Input: part model. Units: mm. Frame: model coordinates. A direction names the side the tool comes from. Coordinates: 2 decimals unless noted, no trailing zeros. Write each loop counter-clockwise with the first axis right and the second up, starting at its lowest first coordinate (ties: lowest second). Pieces come first, ordered by that corner, then holes. Notation, with made-up numbers: (89, 2) - (101, 2) arc R13 cw to (101, 17) - close; hole circle Ø6 at (-1, 23). An arc over 180 degrees is marked (long way). Put each result on its own line as item: value. Start each with the question number.
1. Cut plane C-C, the plane y = 0. Count the separate pieces of the cut face and the enclosed holes in it, and give its area (3 significant figures).
2. Access query for faces 1 (the cylindrical face through (23.82, -1.53, 8.77)), 2 (the flat face through (-16, 0, 17.78)), 3 (the cylindrical face through (12.114, 3.815, 28.4)), 4 (the flat face through (-43, 12.7, 13)). Directions: +Z, -Z, +X, -X, +Y, -Y. A direction counts if a zero-diameter tool reaches every point of the face in a straight line with its end or side. Return the directions, or none.
3. Pull-direction query (X, two-part tool) for faces 5 (the cylindrical face through (0.372, 25.397, 12.878)), 6 (the flat face through (-42, 10.16, 13)), 7 (the flat face through (0, 8.89, 11)); classes: released by +X, released by -X, zero draft, split by the parting line, or undercut.
4. Pin query (flat end, axial travel): pin 1 (10 mm diameter, centred on x = -37.5, y = 2.5, fed in from +Z); pin 2 (1.5 mm diameter, centred on x = 10.5, z = 9.5, fed in from -Y); pin 3 (2 mm diameter, centred on x = 42, y = -0.5, fed in from -Z); pin 4 (12 mm diameter, centred on y = 0.5, z = 7.5, fed in from +X). Return the tip coordinate at first contact, or that it passes through.
5. Cut plane D-D, the plane y = 7. Return loops of the section in (x, z).
6. Line query: line 1 (Y direction, x = 0, z = 19); line 2 (Y direction, x = -41, z = 9); line 3 (X direction, y = 0, z = 25). Output: solid intervals per line, ascending.
7. Cut plane B-B, the plane x = 0. Return loops of the section in (y, z), and give its area (3 significant figures).
8. Cut plane A-A, the plane z = 5. Return loops of the section in (x, y), and give its area (3 significant figures).
from build123d import *

# Parameters (mm, degrees)
F0_W      = 127
F0_H      = 25.4
F1_DEPTH  = 25.4
F2_T      = -2.54
F3_R      = 25.4
F4_DEPTH  = 25.4
F5_R      = 19.05
F6_DEPTH  = 12.7
F7_R      = 12.7
F8_DEPTH  = 25.4
F9_W      = 17.78
F9_H      = 17.78
F10_DEPTH = 150.622
F11_W     = 40.64
F11_H     = 10.16
F12_DEPTH = 12.7
F13_R     = 5.528236
F13_R_2   = 5.08
F14_DEPTH = 17.78


with BuildPart() as f1:
    # F0 (on Top) → F1 (new body)
    with BuildSketch(Plane.XY):
        Rectangle(F0_W, F0_H)
    extrude(amount=F1_DEPTH)

    # F2
    f2_openings = [f1.faces().sort_by_distance(p)[0] for p in [
        (63.5, 0, 12.7),
    ]]
    offset(amount=F2_T, openings=f2_openings)

    # F3 (on face) → F4 (join)
    with BuildSketch(Plane.XY.offset(25.4)):
        Circle(F3_R)
    extrude(amount=-F4_DEPTH)

    # F5 (on face) → F6 (join)
    with BuildSketch(Plane.XY.offset(25.4)):
        Circle(F5_R)
    extrude(amount=F6_DEPTH)

    # F7 (on face) → F8 (cut)
    with BuildSketch(Plane.XY.offset(38.1)):
        Circle(F7_R)
    extrude(amount=-F8_DEPTH, mode=Mode.SUBTRACT)

    # F9 (on face) → F10 (cut)
    with BuildSketch(Plane(origin=(-63.5, 0, 0), x_dir=(0, -1, 0), z_dir=(-1, 0, 0))):
        with Locations((0, 12.7)):
            Rectangle(F9_W, F9_H)
    extrude(amount=-F10_DEPTH, mode=Mode.SUBTRACT)

    # F11 (on face) → F12 (cut)
    with BuildSketch(Plane(origin=(0, 0, 0), x_dir=(1, 0, 0), z_dir=(0, 0, -1))):
        with Locations((-36.008236, 0)):
            Rectangle(F11_W, F11_H)
        with Locations((39.295297, 0)):
            Rectangle(F11_W, F11_H)
    extrude(amount=-F12_DEPTH, mode=Mode.SUBTRACT)

    # F13 (on face) → F14 (join)
    with BuildSketch(Plane(origin=(0, 0, 0), x_dir=(1, 0, 0), z_dir=(0, 0, -1))):
        with Locations((-15.688236, 0)):
            Circle(F13_R)
        with Locations((18.975297, 0)):
            Circle(F13_R_2)
    extrude(amount=-F14_DEPTH)


solid = f1.part
Report:
1. separate pieces: 5
1. enclosed holes: 0
1. area: 955 mm^2
2. face 1: none
2. face 2: +X, -X
2. face 3: +Z
2. face 4: +Z, -Z, -X, +Y
3. face 5: split by the parting line
3. face 6: undercut
3. face 7: zero draft
4. pin 1: stops at z = 25.4
4. pin 2: stops at y = -23.45
4. pin 3: stops at z = 22.86
4. pin 4: stops at x = 63.5
5. outline: (-63.5, 0) - (63.5, 0) - (63.5, 2.54) - (24.42, 2.54) - (24.42, 3.81) - (-24.42, 3.81) - (-24.42, 2.54) - (-60.96, 2.54) - (-60.96, 3.81) - (-63.5, 3.81) - close; (-63.5, 21.59) - (-60.96, 21.59) - (-60.96, 22.86) - (-24.42, 22.86) - (-24.42, 21.59) - (-10.6, 21.59) - (-10.6, 38.1) - (-17.72, 38.1) - (-17.72, 25.4) - (-63.5, 25.4) - close; (10.6, 21.59) - (24.42, 21.59) - (24.42, 22.86) - (63.5, 22.86) - (63.5, 25.4) - (17.72, 25.4) - (17.72, 38.1) - (10.6, 38.1) - close
6. line 1: y = -25.4 to -12.7, 12.7 to 25.4
6. line 2: y = -12.7 to -10.16, 10.16 to 12.7
6. line 3: x = -63.5 to -12.7, 12.7 to 63.5
7. outline: (-25.4, 0) - (25.4, 0) - (25.4, 25.4) - (19.05, 25.4) - (19.05, 38.1) - (12.7, 38.1) - (12.7, 12.7) - (8.89, 12.7) - (8.89, 3.81) - (-8.89, 3.81) - (-8.89, 12.7) - (-12.7, 12.7) - (-12.7, 38.1) - (-19.05, 38.1) - (-19.05, 25.4) - (-25.4, 25.4) - close
7. area: 971 mm^2
8. outline: (-63.5, -12.7) - (-22, -12.7) arc R25.4 ccw to (22, -12.7) - (63.5, -12.7) - (63.5, -10.16) - (23.28, -10.16) arc R25.4 ccw to (23.79, -8.89) - (-23.79, -8.89) arc R25.4 ccw to (-23.28, -10.16) - (-60.96, -10.16) - (-60.96, -8.89) - (-63.5, -8.89) - close; (-63.5, 8.89) - (-60.96, 8.89) - (-60.96, 10.16) - (-23.28, 10.16) arc R25.4 ccw to (-23.79, 8.89) - (23.79, 8.89) arc R25.4 ccw to (23.28, 10.16) - (63.5, 10.16) - (63.5, 12.7) - (22, 12.7) arc R25.4 ccw to (-22, 12.7) - (-63.5, 12.7) - close; circle Ø11.06 at (-15.69, 0); circle Ø10.16 at (18.98, 0)
8. area: 1,740 mm^2
